Geometry check sheet. Reference: the model listing, model coordinates, mm. Round coordinates to 2 decimals unless told otherwise and drop trailing zeros. Write each loop counter-clockwise with the first axis right and the second up, starting at its lowest first coordinate (ties: lowest second). Pieces come first, ordered by that corner, then holes. Notation, with made-up numbers: (81.5, 49.5) -> (85.5, 49.5) arc R28 ccw to (85.5, 77.5) -> close; hole circle Ø10 at (71.25, 43.5). An arc over 180 degrees is marked (long way). Use a Markdown table: item, result.
```python
from build123d import *

# Parameters (mm, degrees)
SKETCH1_W           = 15.3
SKETCH1_H           = 28
SKETCH1_R           = 1.75
SKETCH1_R_2         = 0.5
BOSS_EXTRUDE1_DEPTH = 1
SKETCH2_W           = 4
SKETCH2_H           = 4
BOSS_EXTRUDE2_DEPTH = 1


with BuildPart() as part:
    # Sketch1 → Boss-Extrude1 (new body)
    with BuildSketch(Plane(origin=(0, 0, 0), x_dir=(1, 0, 0), z_dir=(0, 1, 0))):
        with Locations((-1.35, 0)):
            Rectangle(SKETCH1_W, SKETCH1_H)
        with Locations(Location((3.8, 11.5, 0), (0, 0, 270))):
            Circle(SKETCH1_R, mode=Mode.SUBTRACT)
        with Locations(Location((3.8, -11.5, 0), (0, 0, 90))):
            Circle(SKETCH1_R, mode=Mode.SUBTRACT)
        with Locations(Location((-7.65, 0, 0), (0, 0, 270))):
            Circle(SKETCH1_R_2, mode=Mode.SUBTRACT)
        with Locations(Location((-7.65, 2.54, 0), (0, 0, 270))):
            Circle(SKETCH1_R_2, mode=Mode.SUBTRACT)
        with Locations(Location((-7.65, 5.08, 0), (0, 0, 270))):
            Circle(SKETCH1_R_2, mode=Mode.SUBTRACT)
        with Locations(Location((-7.65, 7.62, 0), (0, 0, 270))):
            Circle(SKETCH1_R_2, mode=Mode.SUBTRACT)
        with Locations(Location((-7.65, 10.16, 0), (0, 0, 270))):
            Circle(SKETCH1_R_2, mode=Mode.SUBTRACT)
        with Locations(Location((-7.65, 12.7, 0), (0, 0, 270))):
            Circle(SKETCH1_R_2, mode=Mode.SUBTRACT)
        with Locations(Location((-7.65, -12.7, 0), (0, 0, 90))):
            Circle(SKETCH1_R_2, mode=Mode.SUBTRACT)
        with Locations(Location((-7.65, -10.16, 0), (0, 0, 90))):
            Circle(SKETCH1_R_2, mode=Mode.SUBTRACT)
        with Locations(Location((-7.65, -7.62, 0), (0, 0, 90))):
            Circle(SKETCH1_R_2, mode=Mode.SUBTRACT)
        with Locations(Location((-7.65, -5.08, 0), (0, 0, 90))):
            Circle(SKETCH1_R_2, mode=Mode.SUBTRACT)
        with Locations(Location((-7.65, -2.54, 0), (0, 0, 90))):
            Circle(SKETCH1_R_2, mode=Mode.SUBTRACT)
    extrude(amount=BOSS_EXTRUDE1_DEPTH)

    # Sketch2 → Boss-Extrude2 (add)
    with BuildSketch(Plane(origin=(0, 1, 0), x_dir=(1, 0, 0), z_dir=(0, 1, 0))):
        Rectangle(SKETCH2_W, SKETCH2_H)
    extrude(amount=BOSS_EXTRUDE2_DEPTH)


solid = part.part
```
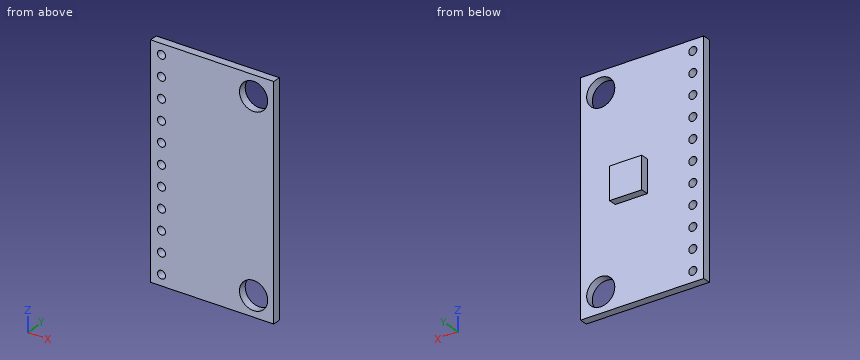
(1) Thickness scan on line 1 (X direction, y = 0.35, z = 10.16); line 2 (X direction, y = 0.4, z = -5.08); line 3 (Z direction, x = 4.75, y = 0.5). Record the ranges inside material, lowest first.
A:
| item | result |
|---|---|
| line 1 | x = -9 to -8.15, -7.15 to 2.67, 4.93 to 6.3 |
| line 2 | x = -9 to -8.15, -7.15 to 6.3 |
| line 3 | z = -14 to -12.97, -10.03 to 10.03, 12.97 to 14 |
(2) Section check B-B on x = 3.8. Record the cut outline in (y, z).
A:
| item | result |
|---|---|
| outline | (0, -14) -> (1, -14) -> (1, -13.25) -> (0, -13.25) -> close; (0, -9.75) -> (1, -9.75) -> (1, 9.75) -> (0, 9.75) -> close; (0, 13.25) -> (1, 13.25) -> (1, 14) -> (0, 14) -> close |
(3) Gauge pin test, flat ends, axial feed: pin 1 Ø2 at (x, z) = (-7, -10.5) entering from +Y; pin 2 Ø1.1 at (y, z) = (1.5, 1) entering from +X; pin 3 Ø0.8 at (y, z) = (1.5, 0.5) entering from -X; pin 4 Ø0.5 at (x, y) = (0, 1.5) entering from +Z. Record the tip position at first contact, or that the pin passes through.
A:
| item | result |
|---|---|
| pin 1 | stops at y = 1 |
| pin 2 | stops at x = 6.3 |
| pin 3 | stops at x = -2 |
| pin 4 | stops at z = 2 |
(4) Section check C-C on y = 0.6. State how many separate pieces and enclosed holes the cut face has, plus the area to 3 significant figures.
A:
| item | result |
|---|---|
| separate pieces | 1 |
| enclosed holes | 13 |
| area | 401 mm2 |
(5) Section check D-D on z = -11.5. Record the cut outline in (x, y), plus the area to 3 significant figures.
A:
| item | result |
|---|---|
| outline | (-9, 0) -> (2.05, 0) -> (2.05, 1) -> (-9, 1) -> close; (5.55, 0) -> (6.3, 0) -> (6.3, 1) -> (5.55, 1) -> close |
| area | 11.8 mm2 |
(6) Section check A-A on z = 0. Record the cut outline in (x, y).
A:
| item | result |
|---|---|
| outline | (-9, 0) -> (-8.15, 0) -> (-8.15, 1) -> (-9, 1) -> close; (-7.15, 0) -> (6.3, 0) -> (6.3, 1) -> (2, 1) -> (2, 2) -> (-2, 2) -> (-2, 1) -> (-7.15, 1) -> close |
